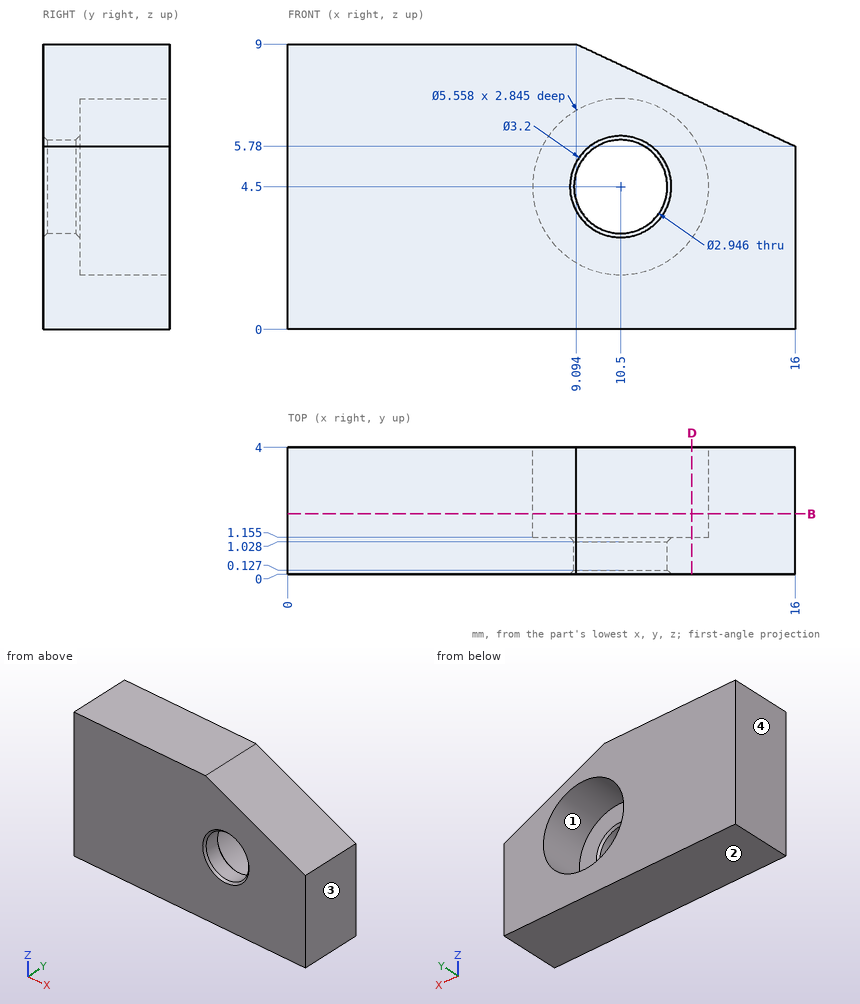
Study the drawing (mm; zero at the part's minimum x, y, z) and answer. Round coordinates to 2 decimals unless told otherwise and drop trailing zeros. Loops run counter-clockwise (first coordinate to the right, second up) from the corner with the lowest first, then second, coordinate; pieces in that order, holes last. Notation, with made-up numbers: (-32, -6.5) -> (0, -6.5) arc R26 cw to (0, 7.5) -> close; hole circle Ø6 at (21.5, 25). An arc over 180 degrees is marked (long way). Write each question's results on one line, items separated by ' | '. Start each with the question number.
1. Section B-B (y = 1.9) is taken. Determine the outline of the cut face in (x, z), plus the area to 3 significant figures.
2. Given pin 1 Ø4.5 at (x, z) = (10.5, 4.5) entering from +Y (1 decimal); pin 2 Ø2.5 at (x, z) = (10.5, 4.5) entering from -Y, each flat-ended and moving along its own axis, determine where each tip first touches the part or whether it passes through.
3. Section D-D (x = 12.75) is taken. Determine the outline of the cut face in (y, z) (1 decimal), plus the area to 3 significant figures.
4. For a pull along X with two mould halves and no side action, classify the marked faces 1, 2, 3 and 4 as +X half, -X half, draft (parallel to the pull), parting line (faces both ways), or undercut.
5. Find the intervals of material crossed by probe 1 along X at (y, z) = (2.9, 4.5); probe 2 along X at (y, z) = (0.45, 4.5); probe 3 along Z at (x, y) = (10.5, 0.75) (1 decimal), in increasing order. Write a range as from..to.
Evaluation:
1) outline: (0, 0) -> (16, 0) -> (16, 5.78) -> (9.09, 9) -> (0, 9) -> close; hole circle Ø5.56 at (10.5, 4.5) | area: 109 mm2
2) pin 1: stops at y = 1.2 | pin 2: passes through
3) outline: (0, 0) -> (4, 0) -> (4, 2.9) -> (1.2, 2.9) -> (1.2, 6.1) -> (4, 6.1) -> (4, 7.3) -> (0, 7.3) -> close | area: 19.9 mm2
4) face 1: undercut | face 2: draft | face 3: +X half | face 4: -X half
5) probe 1: x = 0..7.72, 13.28..16 | probe 2: x = 0..9.03, 11.97..16 | probe 3: z = 0..3, 6..8.3
